Geometry: final body of the model. Coordinates: model frame, mm. A direction names the side the tool comes from. Give positions to 0.01 mm unless a question says otherwise; leave off trailing zeros. Write each loop counter-clockwise with the first axis right and the second up, starting at its lowest first coordinate (ties: lowest second). Pieces come first, ordered by that corner, then holes. Notation, with made-up numbers: (88, -32) -> (126, -32) arc R26 cw to (126, 6) -> close; hole circle Ø9 at (-32.75, -16). An arc over 180 degrees is marked (long way). Answer as a JSON object with one key per item and string values. Group by question number.
(1) Material intervals for probe 1 along Y at (x, z) = (0, -2); probe 2 along X at (y, z) = (-2, -12.5); probe 3 along Z at (x, y) = (-21, -8.5), sorted ascending.
(2) Contact query for flat-ended pins moving along their axis: pin 1 Ø3 at (x, y) = (1.5, -3) entering from -Z; pin 2 Ø2 at (y, z) = (-2, -14) entering from -X; pin 3 Ø1 at (y, z) = (-2, -17) entering from +X; pin 4 Ø2 at (x, y) = (0, 0.5) entering from +Z. Output: stop coordinate, or through.
(3) Section query A-A on z = -34.5. Output: boundary loops of the cut face in (x, y).
(4) Set-up query: faces 5 (the face through (-31, 2.5, -21)), 6 (the face through (6.999, 0.746, 3.521)), 7 (the face through (-19.257, -1.126, 0.07)), 8 (the face through (-18, -6, -13.5)), 9 (the face through (-24, -2, -7)). Return all of +Z, -Z, +X, -X, +Y, -Y with unobstructed straight access to the full face (end or side cutting, diameter ignored); none if empty.
(5) Draft query along Y for faces 1 (the face through (-3.233, -1.341, -2.31)), 2 (the face through (-18, -4, -20)), 3 (the face through (-15.78, -2.27, -7.69)), 4 (the face through (-1.504, -5.219, 3.521)). Return one class per face: +Y half, -Y half, draft (parallel to the pull), parting line (faces both ways), or undercut.
from build123d import *

# Parameters (mm, degrees)
SKETCH1_R                     = 9
BOSS_EXTRUDE1_DEPTH           = 5
SKETCH2_R                     = 7
BOSS_EXTRUDE2_DEPTH           = 1.5
BOSS_EXTRUDE2_TAPER           = 30
BOSS_EXTRUDE2_OTHER_WAY_DEPTH = 1.5
BOSS_EXTRUDE2_OTHER_WAY_TAPER = 30
CUT_EXTRUDE1_DEPTH            = 3
BOSS_EXTRUDE3_DEPTH           = 40
SKETCH5_W                     = 12
SKETCH5_H                     = 23
CUT_EXTRUDE2_DEPTH            = 40
BOSS_EXTRUDE4_DEPTH           = 3.5
SKETCH7_R                     = 2
BOSS_EXTRUDE5_DEPTH           = 3
SKETCH8_R                     = 3.5
CUT_EXTRUDE3_DEPTH            = 53.803882433
BOSS_EXTRUDE6_DEPTH           = 3.5
SKETCH10_R                    = 2.45
BOSS_EXTRUDE7_DEPTH           = 3.5
BOSS_EXTRUDE8_DEPTH           = 3.5
FILLET1_START                 = -26.84
FILLET1_DEPTH                 = 2.84
FILLET1_START_2               = -12
FILLET1_2_DEPTH               = 2.83
FILLET1_START_3               = -26
FILLET1_3_DEPTH               = 21
FILLET1_START_4               = -27.84
FILLET1_4_DEPTH               = 1


with BuildPart() as part:
    # Sketch1 → Boss-Extrude1 (new, symmetric)
    with BuildSketch(Plane.XY):
        Circle(SKETCH1_R)
        with BuildLine():
            Line((-35, -9), (0, -9))
            ThreePointArc((0, -9), (-8.437416666, -3.132091953), (-5.872614409, 6.82))
            ThreePointArc((-5.872614409, 6.82), (-19.465199243, -1.204217751), (-35, -4))
            Line((-35, -4), (-35, -9))
        make_face()
    extrude(amount=BOSS_EXTRUDE1_DEPTH, both=True)

    # Sketch2 → Boss-Extrude2 (add)
    with BuildSketch(Plane(origin=(0, 0, -5), x_dir=(-1, 0, 0), z_dir=(0, 0, -1))):
        Circle(SKETCH2_R)
    extrude(amount=BOSS_EXTRUDE2_DEPTH, taper=BOSS_EXTRUDE2_TAPER)

    # Sketch2 → Boss-Extrude2 other way (add)
    with BuildSketch(Plane(origin=(0, 0, -5), x_dir=(-1, 0, 0), z_dir=(0, 0, -1))):
        Circle(SKETCH2_R)
    extrude(amount=-BOSS_EXTRUDE2_OTHER_WAY_DEPTH, taper=BOSS_EXTRUDE2_OTHER_WAY_TAPER)

    # Sketch3 → Cut-Extrude1 (cut)
    with BuildSketch(Plane.XY.offset(5)):
        with BuildLine():
            Line((1.2, -6.33), (1.8, -4.1378116))
            ThreePointArc((1.8, -4.1378116), (2.058560194, -3.569045514), (2.48, -3.1078116))
            ThreePointArc((2.48, -3.1078116), (2.641475661, -2.955390865), (2.794244497, -2.794244497))
            ThreePointArc((2.794244497, -2.794244497), (2.955390865, -2.641475661), (3.1078116, -2.48))
            ThreePointArc((3.1078116, -2.48), (3.569045514, -2.058560194), (4.1378116, -1.8))
            Line((4.1378116, -1.8), (6.33, -1.2))
            ThreePointArc((6.33, -1.2), (6.992020752, -0.754882576), (7.25, 0))
            ThreePointArc((7.25, 0), (6.992020752, 0.754882576), (6.33, 1.2))
            Line((6.33, 1.2), (4.1378116, 1.8))
            ThreePointArc((4.1378116, 1.8), (3.569045514, 2.058560194), (3.1078116, 2.48))
            ThreePointArc((3.1078116, 2.48), (2.955390865, 2.641475661), (2.794244497, 2.794244497))
            ThreePointArc((2.794244497, 2.794244497), (2.641475661, 2.955390865), (2.48, 3.1078116))
            ThreePointArc((2.48, 3.1078116), (2.058560194, 3.569045514), (1.8, 4.1378116))
            Line((1.8, 4.1378116), (1.2, 6.33))
            ThreePointArc((1.2, 6.33), (0.754882576, 6.992020752), (0, 7.25))
            ThreePointArc((0, 7.25), (-0.754882576, 6.992020752), (-1.2, 6.33))
            Line((-1.2, 6.33), (-1.8, 4.1378116))
            ThreePointArc((-1.8, 4.1378116), (-2.058560194, 3.569045514), (-2.48, 3.1078116))
            ThreePointArc((-2.48, 3.1078116), (-2.641475661, 2.955390865), (-2.794244497, 2.794244497))
            ThreePointArc((-2.794244497, 2.794244497), (-2.955390865, 2.641475661), (-3.1078116, 2.48))
            ThreePointArc((-3.1078116, 2.48), (-3.569045514, 2.058560194), (-4.1378116, 1.8))
            Line((-4.1378116, 1.8), (-6.33, 1.2))
            ThreePointArc((-6.33, 1.2), (-6.992020752, 0.754882576), (-7.25, 0))
            ThreePointArc((-7.25, 0), (-6.992020752, -0.754882576), (-6.33, -1.2))
            Line((-6.33, -1.2), (-4.1378116, -1.8))
            ThreePointArc((-4.1378116, -1.8), (-3.569045514, -2.058560194), (-3.1078116, -2.48))
            ThreePointArc((-3.1078116, -2.48), (-2.955390865, -2.641475661), (-2.794244497, -2.794244497))
            ThreePointArc((-2.794244497, -2.794244497), (-2.641475661, -2.955390865), (-2.48, -3.1078116))
            ThreePointArc((-2.48, -3.1078116), (-2.058560194, -3.569045514), (-1.8, -4.1378116))
            Line((-1.8, -4.1378116), (-1.2, -6.33))
            ThreePointArc((-1.2, -6.33), (-0.754882576, -6.992020752), (0, -7.25))
            ThreePointArc((0, -7.25), (0.754882576, -6.992020752), (1.2, -6.33))
        make_face()
    extrude(amount=-CUT_EXTRUDE1_DEPTH, mode=Mode.SUBTRACT)

    # Sketch4 → Boss-Extrude3 (add)
    with BuildSketch(Plane(origin=(0, 0, -5), x_dir=(-1, 0, 0), z_dir=(0, 0, -1))):
        with BuildLine():
            Line((35, -9), (35, -4))
            Line((35, -4), (9.17, -4))
            ThreePointArc((9.17, -4), (7.844486312, -6.205642902), (6, -8))
            Line((6, -8), (6, -9))
            Line((6, -9), (35, -9))
        make_face()
    extrude(amount=BOSS_EXTRUDE3_DEPTH)

    # Sketch5 → Cut-Extrude2 (cut)
    with BuildSketch(Plane(origin=(0, -4, 0), x_dir=(1, 0, 0), z_dir=(0, 1, 0))):
        with Locations((-18, 25)):
            Rectangle(SKETCH5_W, SKETCH5_H)
    extrude(amount=-CUT_EXTRUDE2_DEPTH, mode=Mode.SUBTRACT)

    # Sketch6 → Boss-Extrude4 (add)
    with BuildSketch(Plane(origin=(0, -4, 0), x_dir=(1, 0, 0), z_dir=(0, 1, 0))):
        with BuildLine():
            Line((-28.5, 29), (-28.5, 21))
            ThreePointArc((-28.5, 21), (-31.5, 18), (-34.5, 21))
            Line((-34.5, 21), (-34.5, 29))
            ThreePointArc((-34.5, 29), (-31.5, 32), (-28.5, 29))
        make_face()
    extrude(amount=BOSS_EXTRUDE4_DEPTH)

    # Sketch7 → Boss-Extrude5 (add)
    with BuildSketch(Plane(origin=(0, -0.5, 0), x_dir=(1, 0, 0), z_dir=(0, 1, 0))):
        with Locations(Location((-31.5, 29, 0), (0, 0, 180))):
            Circle(SKETCH7_R)
        with Locations(Location((-31.5, 21, 0), (0, 0, 180))):
            Circle(SKETCH7_R)
    extrude(amount=BOSS_EXTRUDE5_DEPTH)

    # Sketch8 → Cut-Extrude3 (cut, through all)
    with BuildSketch(Plane(origin=(0, 0, -6.5), x_dir=(-1, 0, 0), z_dir=(0, 0, -1))):
        Circle(SKETCH8_R)
    extrude(amount=-CUT_EXTRUDE3_DEPTH, mode=Mode.SUBTRACT)

    # Sketch9 → Boss-Extrude6 (add)
    with BuildSketch(Plane(origin=(0, -4, 0), x_dir=(1, 0, 0), z_dir=(0, 1, 0))):
        with BuildLine():
            Line((-26.84, 5), (-26.84, 25))
            Line((-26.84, 25), (-21.01, 25))
            ThreePointArc((-21.01, 25), (-18.01, 22), (-15.01, 25))
            Line((-15.01, 25), (-9.17, 25))
            Line((-9.17, 25), (-9.17, 5))
            Line((-9.17, 5), (-12, 5))
            Line((-12, 5), (-12, 8.75))
            ThreePointArc((-12, 8.75), (-11.25, 9.5), (-12, 10.25))
            Line((-12, 10.25), (-12, 16))
            Line((-12, 16), (-17.99, 16))
            Line((-17.99, 16), (-18.01, 16))
            Line((-18.01, 16), (-24, 16))
            Line((-24, 16), (-24, 10.25))
            ThreePointArc((-24, 10.25), (-24.75, 9.5), (-24, 8.75))
            Line((-24, 8.75), (-24, 5))
            Line((-24, 5), (-26.84, 5))
        make_face()
    extrude(amount=BOSS_EXTRUDE6_DEPTH)

    # Sketch10 → Boss-Extrude7 (add)
    with BuildSketch(Plane(origin=(0, -0.5, 0), x_dir=(1, 0, 0), z_dir=(0, 1, 0))):
        with Locations(Location((-18.005833333, 19.5, 0), (0, 0, 180))):
            Circle(SKETCH10_R)
    extrude(amount=BOSS_EXTRUDE7_DEPTH)

    # Sketch11 → Boss-Extrude8 (add)
    with BuildSketch(Plane(origin=(0, -4, 0), x_dir=(1, 0, 0), z_dir=(0, 1, 0))):
        Polygon((-20.68, 9.27091935), (-23.5, 9.27091935), (-21.5, 12.07091935), (-18.05, 8.62091935), (-18, 8.62091935), (-17.95, 8.62091935), (-14.5, 12.07091935), (-12.5, 9.27091935), (-15.32, 9.27091935), (-16.25, 6.07091935), (-17.97, 8.52091935), (-18.03, 8.52091935), (-19.75, 6.07091935), align=None)
    extrude(amount=BOSS_EXTRUDE8_DEPTH)

    # Fillet1: read off the stored shape, not the designer's step
    # Fillet1 outline → Fillet1 (add)
    with BuildSketch(Plane.YZ.offset(FILLET1_START)):
        with BuildLine():
            ThreePointArc((-4, -26), (-3.707106781, -25.292893219), (-3, -25))
            Line((-3, -25), (-4, -25))
            Line((-4, -25), (-4, -26))
        make_face()
    extrude(amount=FILLET1_DEPTH)

    # Fillet1 2 outline → Fillet1 2 (add)
    with BuildSketch(Plane.YZ.offset(FILLET1_START_2)):
        with BuildLine():
            ThreePointArc((-4, -26), (-3.707106781, -25.292893219), (-3, -25))
            Line((-3, -25), (-4, -25))
            Line((-4, -25), (-4, -26))
        make_face()
    extrude(amount=FILLET1_2_DEPTH)

    # Fillet1 3 outline → Fillet1 3 (add)
    with BuildSketch(Plane.XY.offset(FILLET1_START_3)):
        with BuildLine():
            Line((-26.84, -4), (-26.84, -3))
            ThreePointArc((-26.84, -3), (-27.132893219, -3.707106781), (-27.84, -4))
            Line((-27.84, -4), (-26.84, -4))
        make_face()
    extrude(amount=FILLET1_3_DEPTH)

    # Fillet1 4 outline → Fillet1 4 (cut)
    with BuildSketch(Plane.YZ.offset(FILLET1_START_4)):
        with BuildLine():
            Line((-2, -24.999999999), (-3, -25))
            ThreePointArc((-3, -25), (-3.707106781, -25.292893219), (-4, -26))
            Line((-4, -26), (-2, -26))
            Line((-2, -26), (-2, -24.999999999))
        make_face()
    extrude(amount=FILLET1_4_DEPTH, mode=Mode.SUBTRACT)


solid = part.part
Answer list:
{
 "1": {"probe 1": "-9 to -3.5, 3.5 to 9", "probe 2": "-26.84 to -24, -12 to -9.17", "probe 3": "-45 to -36.5, -13.5 to 5"},
 "2": {"pin 1": "z = -6.5", "pin 2": "x = -26.84", "pin 3": "x = -9.17", "pin 4": "through"},
 "3": {"outline": "(-35, -9) -> (-24, -9) -> (-24, -4) -> (-35, -4) -> close; (-12, -9) -> (-6, -9) -> (-6, -8) arc R10 cw to (-9.17, -4) -> (-12, -4) -> close"},
 "4": {"face 5": "+Z, -Z, -X, +Y", "face 6": "+Z", "face 7": "+Z, -X, +Y", "face 8": "+Y, -Y", "face 9": "+Y"},
 "5": {"face 1": "undercut", "face 2": "-Y half", "face 3": "draft", "face 4": "undercut"}
}
